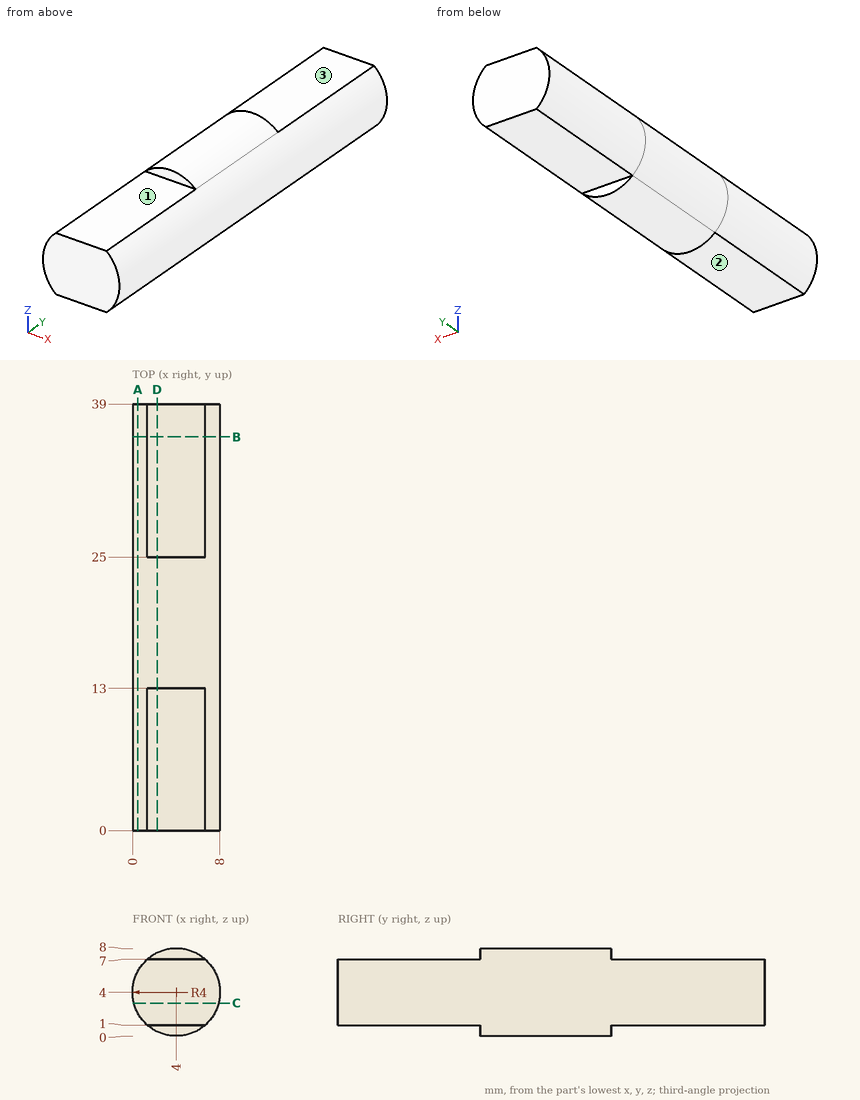
Could you check a few things on this drawing? It's one solid part, dimensions in mm from its lowest x, y, z. A direction names the side the tool comes from. Coordinates: 2 decimals unless noted, no trailing zeros. Loops run counter-clockwise (first coordinate to the right, second up) from the corner with the lowest first, then second, coordinate; pieces in that order, holes last.
1. For the marked faces 1, 2 and 3, which set-ups out of +Z, -Z, +X, -X, +Y, -Y let a thin tool reach every point of the face, with its end or its side?
2. For P1, Ø2, axis at x = 2.5, y = 16, coming from the +Z side; P2, Ø3, axis at x = 6, y = 16.5, coming from the -Z side; P3, Ø1.6, axis at x = 2.5, y = 33.5, coming from the +Z side, each with a flat end and sliding along its axis, tell me the tip position at first contact or that it passes through.
3. Imagine slicing it at D-D (x = 2.25). Please give me the cut outline in (y, z), and give its area (3 significant figures).
4. Imagine slicing it at A-A (x = 0.5). Please give me the cut outline in (y, z), and give its area (3 significant figures).
5. Imagine slicing it at C-C (z = 3). Please give me the cut outline in (x, y), and give its area (3 significant figures).
6. I need wall thicknesses on L1, parallel to Z at x = 1, y = 30; L2, parallel to Z at x = 4.5, y = 6; L3, parallel to X at y = 21.5, z = 3.75. Which ranges of each line are inside material? Lowest first, please.
7. Imagine slicing it at B-B (y = 36). Please give me the cut outline in (x, z).
Computed values:
1. face 1: +Z, +X, -X, -Y
1. face 2: -Z, +X, -X, -Y
1. face 3: +Z, +X, -X, +Y
2. P1: stops at z = 7.97
2. P2: stops at z = 0.03
2. P3: stops at z = 7
3. outline: (0, 1) - (13, 1) - (13, 0.4) - (25, 0.4) - (25, 1) - (39, 1) - (39, 7) - (25, 7) - (25, 7.6) - (13, 7.6) - (13, 7) - (0, 7) - close
3. area: 248 mm2
4. outline: (0, 2.06) - (39, 2.06) - (39, 5.94) - (0, 5.94) - close
4. area: 151 mm2
5. outline: (0.13, 0) - (7.87, 0) - (7.87, 39) - (0.13, 39) - close
5. area: 302 mm2
6. L1: z = 1.35 to 6.65
6. L2: z = 1 to 7
6. L3: x = 0.01 to 7.99
7. outline: (1.35, 1) - (6.65, 1) arc R4 ccw to (6.65, 7) - (1.35, 7) arc R4 ccw to start
